Source: CAD feature listing. Evaluate the final solid. Frame: model axes, mm. Coordinates: 2 decimals unless noted, no trailing zeros. Loops run counter-clockwise (first coordinate to the right, second up) from the corner with the lowest first, then second, coordinate; pieces in that order, holes last.
```python
from build123d import *

# Parameters (mm, degrees)
SKETCH1_W           = 150
SKETCH1_H           = 50
BOSS_EXTRUDE1_DEPTH = 6.35
SKETCH2_R           = 14.225
CUT_EXTRUDE1_DEPTH  = 7.35
SKETCH3_R           = 2.75
CUT_EXTRUDE2_DEPTH  = 7.35


with BuildPart() as part:
    # Sketch1 → Boss-Extrude1 (new body)
    with BuildSketch(Plane.XY):
        with Locations((75, -25)):
            Rectangle(SKETCH1_W, SKETCH1_H)
    extrude(amount=BOSS_EXTRUDE1_DEPTH)

    # Sketch2 → Cut-Extrude1 (cut, through all)
    with BuildSketch(Plane(origin=(0, 0, 0), x_dir=(-1, 0, 0), z_dir=(0, 0, -1))):
        with Locations((-130, -25)):
            Circle(SKETCH2_R)
    extrude(amount=-CUT_EXTRUDE1_DEPTH, mode=Mode.SUBTRACT)

    # Sketch3 → Cut-Extrude2 (cut, through all)
    with BuildSketch(Plane(origin=(0, 0, 0), x_dir=(-1, 0, 0), z_dir=(0, 0, -1))):
        with Locations((-10, -10)):
            Circle(SKETCH3_R)
        with Locations((-10, -40)):
            Circle(SKETCH3_R)
    extrude(amount=-CUT_EXTRUDE2_DEPTH, mode=Mode.SUBTRACT)


solid = part.part
```
Q1. Section query D-D on x = 130. Return the cut outline in (y, z) (3 decimals), then the cut area to 3 significant figures.
Q2. Material intervals for line 1 along Y through (x, z) = (10, 3.5); line 2 along Y through (x, z) = (130, 2.5) (3 decimals); line 3 along X through (y, z) = (-12.5, 1), sorted ascending.
Q3. Section query C-C on z = 1.25. Return the cut outline in (x, y) (3 decimals).
Q4. Section query B-B on y = -25. Return the cut outline in (x, z) (3 decimals), then the cut area to 3 significant figures.
Q5. Section query A-A on x = 10. Return the cut outline in (y, z), then the cut area to 3 significant figures.
Q6. Draft query along Y for faces 1 (the flat face through (74, -50, 3)), 2 (the flat face through (150, -25, 3)), 3 (the cylindrical face through (144.21, -24.37, 3.13)). Return one class per face: released by +Y, released by -Y, zero draft, split by the parting line, or undercut.
Resolved:
1. outline: (-50, 0) - (-39.225, 0) - (-39.225, 6.35) - (-50, 6.35) - close; (-10.775, 0) - (0, 0) - (0, 6.35) - (-10.775, 6.35) - close
1. area: 137 mm2
2. line 1: y = -50 to -42.75, -37.25 to -12.75, -7.25 to 0
2. line 2: y = -50 to -39.225, -10.775 to 0
2. line 3: x = 0 to 8.85, 11.15 to 123.21, 136.79 to 150
3. outline: (0, -50) - (150, -50) - (150, 0) - (0, 0) - close; hole circle Ø5.5 at (10, -40); hole circle Ø5.5 at (10, -10); hole circle Ø28.45 at (130, -25)
4. outline: (0, 0) - (115.775, 0) - (115.775, 6.35) - (0, 6.35) - close; (144.225, 0) - (150, 0) - (150, 6.35) - (144.225, 6.35) - close
4. area: 772 mm2
5. outline: (-50, 0) - (-42.75, 0) - (-42.75, 6.35) - (-50, 6.35) - close; (-37.25, 0) - (-12.75, 0) - (-12.75, 6.35) - (-37.25, 6.35) - close; (-7.25, 0) - (0, 0) - (0, 6.35) - (-7.25, 6.35) - close
5. area: 248 mm2
6. face 1: released by -Y
6. face 2: zero draft
6. face 3: undercut
